Geometry: final body of the model. Coordinates: model frame, mm. A direction names the side the tool comes from. Give positions to 0.01 mm unless a question says otherwise; leave off trailing zeros. Loops run counter-clockwise (first coordinate to the right, second up) from the corner with the lowest first, then second, coordinate; pieces in that order, holes last. Notation, with made-up numbers: (38, 89) - (54, 89) arc R29 ccw to (54, 109) - close; hole circle Ø4 at (74, 85.5). An arc over 180 degrees is marked (long way). Answer in a Markdown table with one row per item.
from build123d import *

# Parameters (mm, degrees)
SKETCH_1_R          = 0.8
EXTRUDE_5_DEPTH     = 5
SKETCH_6_R          = 0.8
CUT_EXTRUDE_1_DEPTH = 1.5
SKETCH_7_R          = 1.5
CUT_EXTRUDE_2_DEPTH = 21.597329924
CUT_EXTRUDE_4_DEPTH = 1.8
SKETCH_9_R          = 1
CUT_EXTRUDE_5_DEPTH = 1
SKETCH_10_W         = 4
SKETCH_10_H         = 1.8
CUT_EXTRUDE_6_DEPTH = 4.6


with BuildPart() as part:
    # ｽｹｯﾁ1 → ﾎﾞｽ - 押し出し5 (new body)
    # profile 1 of 3: a face of its own
    with BuildSketch(Plane.YZ):
        with BuildLine():
            Line((-3, -10.5), (-3, -7.95298686))
            ThreePointArc((-3, -7.95298686), (-8.482257997, -0.548907345), (-4, 7.5))
            Line((-4, 7.5), (-17, 7.5))
            Line((-17, 7.5), (-17, -10.5))
            Line((-17, -10.5), (-3, -10.5))
        make_face()
    # profile 2 of 3: a face of its own
    with BuildSketch(Plane.YZ):
        with BuildLine():
            ThreePointArc((-3, 0), (0, 3), (3, 0))
            Line((3, 0), (3, -7.95298686))
            ThreePointArc((3, -7.95298686), (6.991065727, -4.834769901), (8.5, 0))
            ThreePointArc((8.5, 0), (7.288689869, 4.373213921), (4, 7.5))
            Line((4, 7.5), (-4, 7.5))
            ThreePointArc((-4, 7.5), (-8.482257997, -0.548907345), (-3, -7.95298686))
            Line((-3, -7.95298686), (-3, 0))
        make_face()
        with Locations(Location((-5, -2.886751346, 0), (0, 0, 270))):
            Circle(SKETCH_1_R, mode=Mode.SUBTRACT)
        with Locations(Location((5.074182173, -2.886751346, 0), (0, 0, 270))):
            Circle(SKETCH_1_R, mode=Mode.SUBTRACT)
        with Locations(Location((-5, 2.929580443, 0), (0, 0, 270))):
            Circle(SKETCH_1_R, mode=Mode.SUBTRACT)
        with Locations(Location((5.074182173, 2.929580443, 0), (0, 0, 270))):
            Circle(SKETCH_1_R, mode=Mode.SUBTRACT)
        with Locations(Location((0.037091086, 5.837746338, 0), (0, 0, 270))):
            Circle(SKETCH_1_R, mode=Mode.SUBTRACT)
    # profile 3 of 3: a face of its own
    with BuildSketch(Plane.YZ):
        with BuildLine():
            ThreePointArc((8.5, 0), (6.991065727, -4.834769901), (3, -7.95298686))
            Line((3, -7.95298686), (3, -10.5))
            Line((3, -10.5), (17, -10.5))
            Line((17, -10.5), (17, 7.5))
            Line((17, 7.5), (4, 7.5))
            ThreePointArc((4, 7.5), (7.288689869, 4.373213921), (8.5, 0))
        make_face()
    extrude(amount=-EXTRUDE_5_DEPTH)

    # ｽｹｯﾁ6 → ｶｯﾄ - 押し出し1 (cut)
    # profile 1 of 5: a face of its own
    with BuildSketch(Plane.YZ):
        with BuildLine():
            ThreePointArc((-4, 7.5), (-7.288689869, 4.373213921), (-8.5, 0))
            Line((-8.5, 0), (-3, 0))
            ThreePointArc((-3, 0), (0, 3), (3, 0))
            Line((3, 0), (8.5, 0))
            ThreePointArc((8.5, 0), (7.288689869, 4.373213921), (4, 7.5))
            Line((4, 7.5), (-4, 7.5))
        make_face()
        with Locations(Location((-5, 2.929580443, 0), (0, 0, 270))):
            Circle(SKETCH_6_R, mode=Mode.SUBTRACT)
        with Locations(Location((5.074182173, 2.929580443, 0), (0, 0, 270))):
            Circle(SKETCH_6_R, mode=Mode.SUBTRACT)
        with Locations(Location((0.037091086, 5.837746338, 0), (0, 0, 270))):
            Circle(SKETCH_6_R, mode=Mode.SUBTRACT)
    # profile 2 of 5: a face of its own
    with BuildSketch(Plane.YZ):
        with BuildLine():
            Line((-3, 0), (-8.5, 0))
            ThreePointArc((-8.5, 0), (-6.991065727, -4.834769901), (-3, -7.95298686))
            Line((-3, -7.95298686), (-3, 0))
        make_face()
        with Locations(Location((-5, -2.886751346, 0), (0, 0, 270))):
            Circle(SKETCH_6_R, mode=Mode.SUBTRACT)
    # profile 3 of 5: a face of its own
    with BuildSketch(Plane.YZ):
        with BuildLine():
            Line((8.5, 0), (3, 0))
            Line((3, 0), (3, -7.95298686))
            ThreePointArc((3, -7.95298686), (6.991065727, -4.834769901), (8.5, 0))
        make_face()
        with Locations(Location((5.074182173, -2.886751346, 0), (0, 0, 270))):
            Circle(SKETCH_6_R, mode=Mode.SUBTRACT)
    # profile 4 of 5: a face of its own
    with BuildSketch(Plane.YZ):
        with BuildLine():
            ThreePointArc((8.5, 0), (6.991065727, -4.834769901), (3, -7.95298686))
            Line((3, -7.95298686), (3, -10.5))
            Line((3, -10.5), (8.5, -10.5))
            Line((8.5, -10.5), (8.5, 0))
        make_face()
    # profile 5 of 5: a face of its own
    with BuildSketch(Plane.YZ):
        with BuildLine():
            ThreePointArc((-3, -7.95298686), (-6.991065727, -4.834769901), (-8.5, 0))
            Line((-8.5, 0), (-8.5, -10.5))
            Line((-8.5, -10.5), (-3, -10.5))
            Line((-3, -10.5), (-3, -7.95298686))
        make_face()
    extrude(amount=-CUT_EXTRUDE_1_DEPTH, mode=Mode.SUBTRACT)

    # ｽｹｯﾁ7 → ｶｯﾄ - 押し出し2 (cut, through all)
    with BuildSketch(Plane(origin=(-5, 0, 0), x_dir=(0, -1, 0), z_dir=(-1, 0, 0))):
        with Locations(Location((-13.611024943, -1.95, 0), (0, 0, 90))):
            Circle(SKETCH_7_R)
        with Locations(Location((13.611024943, -1.95, 0), (0, 0, 270))):
            Circle(SKETCH_7_R)
    extrude(amount=-CUT_EXTRUDE_2_DEPTH, mode=Mode.SUBTRACT)

    # ｽｹｯﾁ8 → ｶｯﾄ - 押し出し4 (cut)
    with BuildSketch(Plane.YZ):
        Polygon((10.81922748, -3.513926764), (10.860725904, -0.314195857), (13.652523367, 1.249730908), (16.402822406, -0.386073236), (16.361323982, -3.585804143), (13.569526519, -5.149730908), align=None)
        Polygon((-10.860725904, -0.314195857), (-13.652523367, 1.249730908), (-16.402822406, -0.386073236), (-16.361323982, -3.585804143), (-13.569526519, -5.149730908), (-10.81922748, -3.513926764), align=None)
    extrude(amount=-CUT_EXTRUDE_4_DEPTH, mode=Mode.SUBTRACT)

    # ｽｹｯﾁ9 → ｶｯﾄ - 押し出し5 (cut)
    with BuildSketch(Plane(origin=(0, 0, -10.5), x_dir=(1, 0, 0), z_dir=(0, 0, -1))):
        with Locations(Location((-2.3, 12.508141571, 0), (0, 0, 180))):
            Circle(SKETCH_9_R)
        with Locations((-2.3, -12.508141571)):
            Circle(SKETCH_9_R)
    extrude(amount=-CUT_EXTRUDE_5_DEPTH, mode=Mode.SUBTRACT)

    # ｽｹｯﾁ10 → ｶｯﾄ - 押し出し6 (cut)
    with BuildSketch(Plane.YZ):
        with Locations((-12.5, -8.6)):
            Rectangle(SKETCH_10_W, SKETCH_10_H)
        with Locations((12.5, -8.6)):
            Rectangle(SKETCH_10_W, SKETCH_10_H)
    extrude(amount=-CUT_EXTRUDE_6_DEPTH, mode=Mode.SUBTRACT)


solid = part.part
Q1. Cut plane B-B (z = -1). Output: boundary loops of the cut face in (x, y), and give its area (3 significant figures).
Check values:
| item | result |
|---|---|
| outline | (-5, -17) - (0, -17) - (0, -16.39) - (-1.8, -16.39) - (-1.8, -14.77) - (-5, -14.77) - close; (-5, -12.45) - (-1.8, -12.45) - (-1.8, -10.85) - (0, -10.85) - (0, -8.5) - (-1.5, -8.5) - (-1.5, -3) - (-5, -3) - close; (-5, 3) - (-1.5, 3) - (-1.5, 8.5) - (0, 8.5) - (0, 10.85) - (-1.8, 10.85) - (-1.8, 12.45) - (-5, 12.45) - close; (-5, 14.77) - (-1.8, 14.77) - (-1.8, 16.39) - (0, 16.39) - (0, 17) - (-5, 17) - close |
| area | 88.7 mm² |
Q2. Material intervals for line 1 along Y through (x, z) = (-2.3, -10.25); line 2 along Y through (x, z) = (-0.2, -8); line 3 along Z through (x, y) = (-0.7, -13), sorted ascending.
Check values:
| item | result |
|---|---|
| line 1 | -17 to -13.51, -11.51 to -3, 3 to 11.51, 13.51 to 17 |
| line 2 | -17 to -14.5, -10.5 to -8.5, 8.5 to 10.5, 14.5 to 17 |
| line 3 | -10.5 to -9.5, -7.7 to -4.81, 0.88 to 7.5 |
Q3. First-contact query: pin 1 (6 mm diameter, centred on y = -14, z = -1, fed in from +X); pin 2 (1.2 mm diameter, centred on x = -2, y = 12.5, fed in from -Z). Flat tips, straight axial feed; report the tip coordinate or a pass-through.
Check values:
| item | result |
|---|---|
| pin 1 | x = 0 |
| pin 2 | z = -7.7 |
Q4. Cut plane C-C (y = -5). Output: boundary loops of the cut face in (x, z), and give its area (3 significant figures).
Check values:
| item | result |
|---|---|
| outline | (-5, -10.5) - (-1.5, -10.5) - (-1.5, -3.69) - (-5, -3.69) - close; (-5, -2.09) - (-1.5, -2.09) - (-1.5, 2.13) - (-5, 2.13) - close; (-5, 3.73) - (-1.5, 3.73) - (-1.5, 6.87) - (0, 6.87) - (0, 7.5) - (-5, 7.5) - close |
| area | 52.7 mm² |
Q5. Reachability of faces 4 (the cylindrical face through (-3.226, 4.364, -3.256)), 5 (the flat face through (-3, 3, -5)), 6 (the cylindrical face through (-0.74, 7.32, 4.32)), 7 (the flat face through (-5, -4, -1)), 8 (the flat face through (-0.89, -12.21, -4.34)) from +Z, -Z, +X, -X, +Y, -Y: full face, straight path, thin tool, end or side. Return the list, or none.
Check values:
| item | result |
|---|---|
| face 4 | +X, -X |
| face 5 | -Z, +X, -X |
| face 6 | -Z, +X |
| face 7 | +Z, -Z, -X, +Y, -Y |
| face 8 | +X |
Q6. Draft query along Z for faces 1 (the cylindrical face through (-3.226, 0.072, 6.637)), 2 (the flat face through (-1, 8.5, -5)), 3 (the cylindrical face through (-0.74, -7.255, 4.428)). Return one class per face: pulls with the +Z half, pulls with the -Z half, needs draft (parallel to the pull), parting line crosses it, or undercut.
Check values:
| item | result |
|---|---|
| face 1 | undercut |
| face 2 | needs draft |
| face 3 | pulls with the -Z half |
Q7. Cut plane A-A (x = -2.3). Give the number of separate pieces and of enclosed holes in the cut face, and give its area (3 significant figures).
Check values:
| item | result |
|---|---|
| separate pieces | 1 |
| enclosed holes | 7 |
| area | 492 mm² |
